from build123d import *

# Parameters (mm, degrees)
SKETCH1_W              = 42
SKETCH1_H              = 60
SKETCH1_R              = 3.5
BASE_FLANGE2_DEPTH     = 2
SKETCHED_BEND1_DEPTH   = 42
SKETCHED_BEND1_2_DEPTH = 42


# Read off the part's stored shape, not the designer's step: Sketched Bend1
# Sheet-metal steps are written as plain solids
with BuildPart() as part:
    # Sketch1 → Base-Flange2 (new body)
    with BuildSketch(Plane(origin=(0, 0, 0), x_dir=(1, 0, 0), z_dir=(0, 1, 0))):
        with Locations((21, -30)):
            Rectangle(SKETCH1_W, SKETCH1_H)
        with Locations(Location((21, -10, 0), (0, 0, 270))):
            Circle(SKETCH1_R, mode=Mode.SUBTRACT)
    extrude(amount=-BASE_FLANGE2_DEPTH)

    # Sketched Bend1 outline → Sketched Bend1 (cut)
    with BuildSketch(Plane.YZ):
        with BuildLine():
            ThreePointArc((-2, 18.07), (-1.464101615, 20.07), (0, 21.534101616))
            Line((0, 21.534101616), (0, 60))
            Line((0, 60), (-2, 60))
            Line((-2, 60), (-2, 18.07))
        make_face()
    extrude(amount=SKETCHED_BEND1_DEPTH, mode=Mode.SUBTRACT)

    # Sketched Bend1 2 outline → Sketched Bend1 2 (add)
    with BuildSketch(Plane.YZ):
        with BuildLine():
            ThreePointArc((0, 18.07), (0.585786438, 19.484213562), (2, 20.07))
            Line((2, 20.07), (39.21761102, 20.07))
            Line((39.21761102, 20.07), (39.21761102, 22.07))
            Line((39.21761102, 22.07), (2, 22.07))
            ThreePointArc((2, 22.07), (0.96472382, 21.933703305), (0, 21.534101616))
            Line((0, 21.534101616), (0, 18.07))
        make_face()
    extrude(amount=SKETCHED_BEND1_2_DEPTH)


solid = part.part
Check sheet for the modelled part. Datum: model origin and axes. Units: mm. A direction names the side the tool comes from. Round coordinates to 2 decimals unless told otherwise and drop trailing zeros. Write each loop counter-clockwise with the first axis right and the second up, starting at its lowest first coordinate (ties: lowest second). Pieces come first, ordered by that corner, then holes. Notation, with made-up numbers: (55.25, 72.5) -> (90.25, 72.5) arc R12 ccw to (90.25, 77.5) -> close; hole circle Ø11 at (-34, 4). An arc over 180 degrees is marked (long way). Answer as CSV lines item,"result". Start each with the question number.
1) Tool access check on faces 1 (the flat face through (21, 0, 5)), 2 (the flat face through (0, 14, 21)). Record the directions out of +Z, -Z, +X, -X, +Y, -Y that give a thin tool (end or side, any length) a straight path to the whole face; none if there is none.
2) Section check A-A on x = 21. Enter the section's corners in (y, z), and give its area (3 significant figures).
3) Section check B-B on z = 10. Enter the section's corners in (x, y), and give its area (3 significant figures).
4) Section check D-D on y = 11. Enter the section's corners in (x, z).
5) Release check for a two-part mould opening along Z. For faces 3 (the flat face through (42, 14, 21)), 4 (the flat face through (21, 21, 22.07)), 5 (the flat face through (21, 20, 20.07)), 6 (the cylindrical face through (23.365, -0.986, 7.42)) record: pulls with the +Z half, pulls with the -Z half, needs draft (parallel to the pull), parting line crosses it, or undercut.
6) Go/stop test with flat-tipped pins: P1, Ø1.5, axis at x = 32.5, z = 12.5, coming from the +Y side; P2, Ø5, axis at x = 33.5, y = 3.5, coming from the -Z side; P3, Ø4, axis at y = 4.5, z = 16.5, coming from the +X side. Record where each tip stops, or that it passes through.
7) Section check C-C on x = 30. Enter the section's corners in (y, z).
8) Material ranges on line 1 (X direction, y = -0.95, z = 10); line 2 (Z direction, x = 29, y = 10.5); line 3 (Y direction, x = 12.5, z = 13), recorded low to high. Write a range as from..to.
Found:
1,face 1,"-Z, +X, -X, +Y"
1,face 2,"+Z, -Z, -X, +Y, -Y"
2,outline,"(-2, 0) -> (0, 0) -> (0, 6.5) -> (-2, 6.5) -> close; (-2, 13.5) -> (0, 13.5) -> (0, 18.07) arc R2 cw to (2, 20.07) -> (39.22, 20.07) -> (39.22, 22.07) -> (2, 22.07) arc R4 ccw to (-2, 18.07) -> close"
2,area,"106 mm^2"
3,outline,"(0, -2) -> (17.5, -2) -> (17.5, 0) -> (0, 0) -> close; (24.5, -2) -> (42, -2) -> (42, 0) -> (24.5, 0) -> close"
3,area,"70.0 mm^2"
4,outline,"(0, 20.07) -> (42, 20.07) -> (42, 22.07) -> (0, 22.07) -> close"
5,face 3,"needs draft"
5,face 4,"pulls with the +Z half"
5,face 5,"pulls with the -Z half"
5,face 6,"undercut"
6,P1,"stops at y = 0"
6,P2,"stops at z = 19.8"
6,P3,"passes through"
7,outline,"(-2, 0) -> (0, 0) -> (0, 18.07) arc R2 cw to (2, 20.07) -> (39.22, 20.07) -> (39.22, 22.07) -> (2, 22.07) arc R4 ccw to (-2, 18.07) -> close"
8,line 1,"x = 0..17.5, 24.5..42"
8,line 2,"z = 20.07..22.07"
8,line 3,"y = -2..0"
